```python
from build123d import *

# Parameters (mm, degrees)
EXTRUDE209_DEPTH = 10
EXTRUDE208_DEPTH = 10


with BuildPart() as obj1:
    # Sketch210 → Extrude209 (new body)
    with BuildSketch(Plane.XY.offset(-78)):
        with BuildLine():
            ThreePointArc((81, -8.75), (78.701903, -9.701903), (77.75, -12))
            Line((77.75, -12), (77.75, -14))
            ThreePointArc((77.75, -14), (78.701903, -16.298097), (81, -17.25))
            Line((81, -17.25), (135, -17.25))
            ThreePointArc((135, -17.25), (137.298097, -16.298097), (138.25, -14))
            Line((138.25, -14), (138.25, -12))
            ThreePointArc((138.25, -12), (137.298097, -9.701903), (135, -8.75))
            Line((135, -8.75), (81, -8.75))
        make_face()
    extrude(amount=-EXTRUDE209_DEPTH)


with BuildPart() as wirecuts:
    # Sketch209 → Extrude208 (new body)
    with BuildSketch(Plane.XY.offset(-77.25)):
        with BuildLine():
            ThreePointArc((125.5, -2.18), (123.802944, -2.882944), (123.1, -4.58))
            Line((123.1, -8.75), (123.1, -4.58))
            Line((134.9, -8.75), (123.1, -8.75))
            Line((134.9, -4.58), (134.9, -8.75))
            ThreePointArc((134.9, -4.58), (134.197056, -2.882944), (132.5, -2.18))
            Line((125.5, -2.18), (132.5, -2.18))
        make_face()
    extrude(amount=-EXTRUDE208_DEPTH)

    # Fusion202: union obj1
    add(obj1.part)


solid = wirecuts.part
```
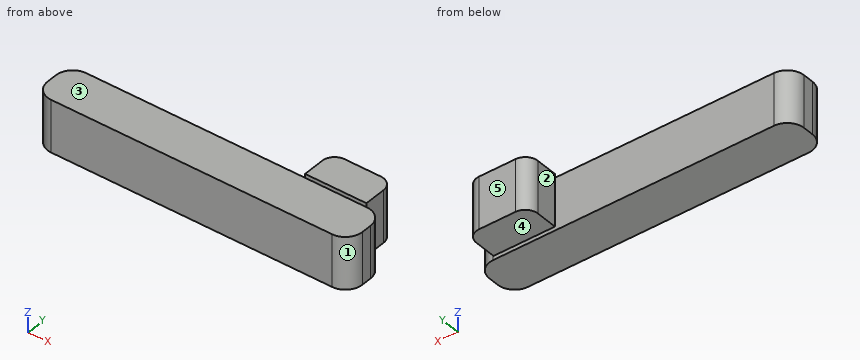
The model under review builds one solid part; all positions refer to its coordinate system, in mm. Face numbers are marked on the shaded views. A direction names the side the tool comes from. Give positions to 0.01 mm unless a question says otherwise; leave off trailing zeros. Write each loop counter-clockwise with the first axis right and the second up, starting at its lowest first coordinate (ties: lowest second). Pieces come first, ordered by that corner, then holes. Notation, with made-up numbers: (15.25, 17) - (50.25, 17) arc R22 cw to (50.25, 27) - close; hole circle Ø3 at (80.25, 69). An arc over 180 degrees is marked (long way). Answer in a Markdown table with one row per item. Add a question column.
1. We need section A-A on z = -80. Write out the cut boundary in (x, y).
2. We need section C-C on y = -13.25. Write out the cut boundary in (x, z).
3. We need section D-D on y = -6. Write out the cut boundary in (x, z).
4. Insertion check: P1, Ø2, axis at y = -6, z = -80.5, coming from the +X side; P2, Ø4.5, axis at x = 121.5, y = -12.5, coming from the +Z side; P3, Ø5, axis at x = 108.5, z = -84.5, coming from the +Y side. Each pin has a flat end and moves straight along its axis. Give the tip position at first contact, or say it passes through.
5. Tool access review of the marked faces 1, 2, 3, 4 and 5: name each direction out of +Z, -Z, +X, -X, +Y, -Y from which nothing blocks a thin tool from reaching the whole face with its end or side.
6. Wall thickness on line 1 along Z through (x, y) = (96, -13.75); line 2 along Y through (x, z) = (83.5, -85.75): over which ranges is each line inside the solid? List them lowest first. Write a range as [from, to].
7. We need section B-B on x = 126.5. Write out the cut boundary in (y, z).
Ans:
| question | item | result |
|---|---|---|
| 1 | outline | (77.75, -14) arc R3.25 ccw to (81, -17.25) - (135, -17.25) arc R3.25 ccw to (138.25, -14) - (138.25, -12) arc R3.25 ccw to (135, -8.75) - (134.9, -8.75) - (134.9, -4.58) arc R2.4 ccw to (132.5, -2.18) - (125.5, -2.18) arc R2.4 ccw to (123.1, -4.58) - (123.1, -8.75) - (81, -8.75) arc R3.25 ccw to (77.75, -12) - close |
| 2 | outline | (77.75, -88) - (138.25, -88) - (138.25, -78) - (77.75, -78) - close |
| 3 | outline | (123.1, -87.25) - (134.9, -87.25) - (134.9, -77.25) - (123.1, -77.25) - close |
| 4 | P1 | stops at x = 134.9 |
| 4 | P2 | stops at z = -78 |
| 4 | P3 | stops at y = -8.75 |
| 5 | face 1 | +Z, -Z, +X, -Y |
| 5 | face 2 | +Z, -Z, -X, +Y |
| 5 | face 3 | +Z, +X, -X, -Y |
| 5 | face 4 | -Z, +X, -X, +Y |
| 5 | face 5 | +Z, -Z, +X, -X, +Y |
| 6 | line 1 | z = [-88, -78] |
| 6 | line 2 | y = [-17.25, -8.75] |
| 7 | outline | (-17.25, -88) - (-8.75, -88) - (-8.75, -87.25) - (-2.18, -87.25) - (-2.18, -77.25) - (-8.75, -77.25) - (-8.75, -78) - (-17.25, -78) - close |
